```python
from build123d import *

# Parameters (mm, degrees)
SKETCH067_R               = 8.5
PAD009_DEPTH              = 9
SKETCH068_W               = 17
SKETCH068_H               = 13
PAD010_DEPTH              = 1
SKETCH069_W               = 2
SKETCH069_H               = 3
PAD011_DEPTH              = 2.5
PAD012_DEPTH              = 21
FUSION002_PLACEMENT_ANGLE = 180


with BuildPart() as body009:
    # Sketch067 → Pad009 (new body)
    with BuildSketch(Plane.XY):
        with Locations((43.911242, 2.762661)):
            Circle(SKETCH067_R)
    extrude(amount=PAD009_DEPTH)

    # Sketch068 → Pad010 (join)
    with BuildSketch(Plane.XY.offset(3)):
        with Locations((43.911242, -3.737339)):
            Rectangle(SKETCH068_W, SKETCH068_H)
    extrude(amount=PAD010_DEPTH)

    # Sketch069 → Pad011 (join)
    with BuildSketch(Plane.XY):
        with Locations((51.911242, 2.762661)):
            Rectangle(SKETCH069_W, SKETCH069_H)
    extrude(amount=-PAD011_DEPTH)


with BuildPart() as pot:
    # Sketch070 → Pad012 (new body)
    with BuildSketch(Plane.XY):
        with BuildLine():
            Line((41.956765, 0.26313), (41.959666, 5.256243))
            ThreePointArc((41.956765, 0.26313), (47.080742, 2.75671), (41.959666, 5.256243))
        make_face()
    extrude(amount=PAD012_DEPTH)


with BuildPart() as pot_1:
    # Body010 placement: moved
    add(pot.part.moved(Location((0, 0, -21))))

    # Fusion002: union Body009
    add(body009.part)


with BuildPart() as pot_2:
    # Fusion002 placement: moved
    add(pot_1.part.moved(Location((88, 0, 14))).rotate(Axis((88, 0, 14), (0, 1, 0)), FUSION002_PLACEMENT_ANGLE))


solid = pot_2.part
```
Check sheet for the modelled part. Datum: model origin and axes. Units: mm. A direction names the side the tool comes from. Round coordinates to 2 decimals unless told otherwise and drop trailing zeros. Loops run counter-clockwise (first coordinate to the right, second up) from the corner with the lowest first, then second, coordinate; pieces in that order, holes last. Notation, with made-up numbers: (64, 35.25) -> (93, 35.25) arc R13 cw to (93, 41.25) -> close; hole circle Ø10 at (23.25, 11). An arc over 180 degrees is marked (long way). Answer in a Markdown table with one row per item.
Q1. Thickness scan on L1, parallel to Z at x = 50.25, y = 8.25; L2, parallel to X at y = 1.5, z = 14.25; L3, parallel to Z at x = 45, y = -8. Record the ranges inside material, lowest first.
Data:
| item | result |
|---|---|
| L1 | z = 5 to 14 |
| L2 | x = 35.09 to 37.09, 41.18 to 46.04 |
| L3 | z = 10 to 11 |
Q2. Release check for a two-part mould opening along X. For faces 1 (the face through (44, 3, 5)), 2 (the face through (45.2, 11.19, 9.56)), 3 (the face through (37.089, 3, 15)), 4 (the face through (35.589, -3.8, 10.5)) record: released by +X, released by -X, zero draft, split by the parting line, or undercut.
Data:
| item | result |
|---|---|
| face 1 | zero draft |
| face 2 | split by the parting line |
| face 3 | undercut |
| face 4 | released by -X |
Q3. Sectioned sample at B-B on x = 51.75. Enter the section's corners in (y, z).
Data:
| item | result |
|---|---|
| outline | (-10.24, 10) -> (-0.92, 10) -> (-0.92, 5) -> (6.44, 5) -> (6.44, 14) -> (-0.92, 14) -> (-0.92, 11) -> (-10.24, 11) -> close |
Q4. Go/stop test with flat-tipped pins: P1, Ø0.8, axis at y = -6, z = 10.5, coming from the -X side; P2, Ø1, axis at x = 36, z = 15.5, coming from the +Y side; P3, Ø4, axis at y = -2.5, z = 15, coming from the +X side; P4, Ø0.7, axis at x = 35.5, y = 3.5, coming from the -Z side. Record where each tip stops, or that it passes through.
Data:
| item | result |
|---|---|
| P1 | stops at x = 35.59 |
| P2 | stops at y = 4.26 |
| P3 | stops at x = 51.82 |
| P4 | stops at z = 5 |
Q5. Sectioned sample at C-C on z = 8.25. Enter the section's corners in (x, y), then the cut area to 3 significant figures.
Data:
| item | result |
|---|---|
| outline | circle Ø17 at (44.09, 2.76) |
| area | 227 mm^2 |
Q6. Set-up check for faces 5 (the face through (44, -7, 10)), 6 (the face through (36, 4.263, 15)), 7 (the face through (40.92, 2.66, 24.65)), 8 (the face through (36, 3, 16.5)): record each of +Z, -Z, +X, -X, +Y, -Y from which the full face is reachable in a straight line by a thin tool's end or side.
Data:
| item | result |
|---|---|
| face 5 | -Z, -Y |
| face 6 | +Z, -X, +Y |
| face 7 | +Z |
| face 8 | +Z, -X, +Y, -Y |
Q7. Sectioned sample at D-D on x = 41.5. Enter the section's corners in (y, z), then the cut area to 3 significant figures.
Data:
| item | result |
|---|---|
| outline | (-10.24, 10) -> (-5.33, 10) -> (-5.33, 5) -> (10.86, 5) -> (10.86, 14) -> (4.59, 14) -> (4.59, 35) -> (0.93, 35) -> (0.93, 14) -> (-5.33, 14) -> (-5.33, 11) -> (-10.24, 11) -> close |
| area | 227 mm^2 |
Q8. Sectioned sample at A-A on y = -2. Enter the section's corners in (x, z), then the cut area to 3 significant figures.
Data:
| item | result |
|---|---|
| outline | (35.59, 10) -> (37.05, 10) -> (37.05, 5) -> (51.13, 5) -> (51.13, 10) -> (52.59, 10) -> (52.59, 11) -> (51.13, 11) -> (51.13, 14) -> (37.05, 14) -> (37.05, 11) -> (35.59, 11) -> close |
| area | 130 mm^2 |
